The drawing under review shows one solid part. Ordinate dimensions are in mm from its lowest x, y, z. A direction names the side the tool comes from. Round coordinates to 2 decimals unless told otherwise and drop trailing zeros. Put each result on its own line as item: value. Start each with the question number.
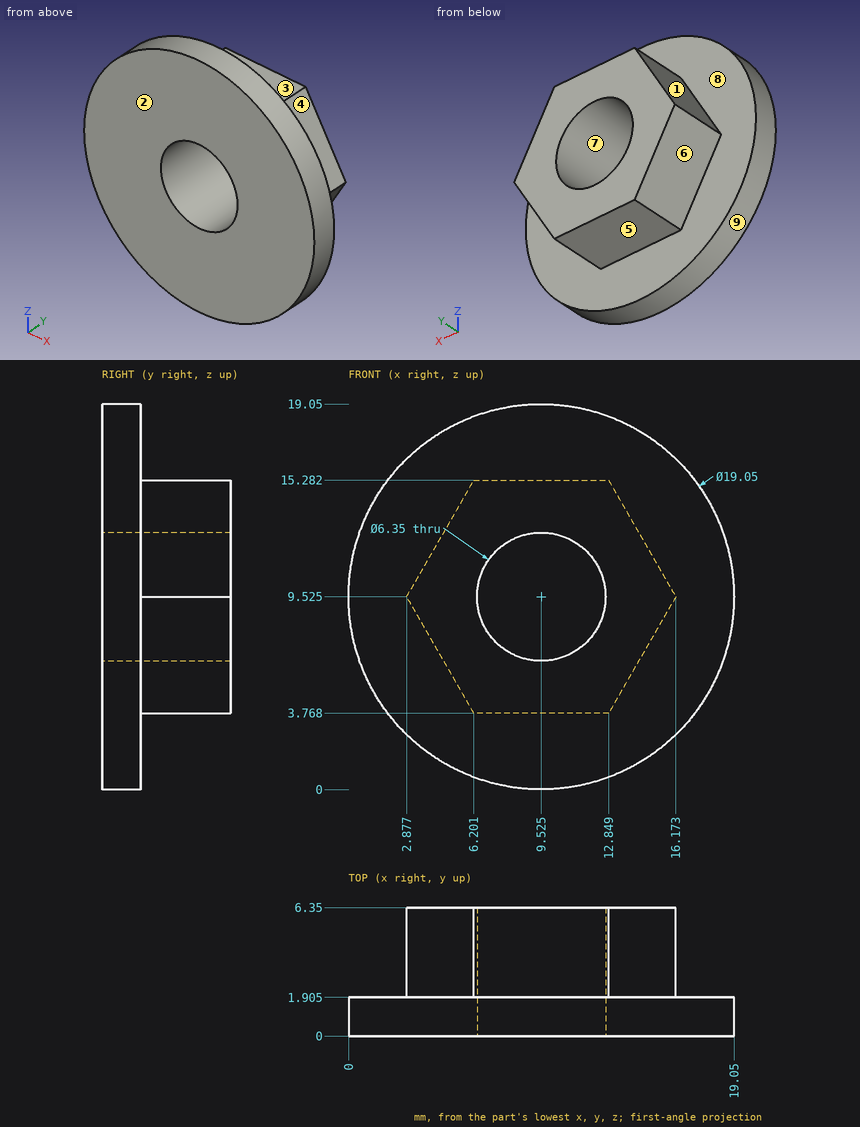
Item 1: For L1, parallel to Y at x = 15.75, z = 3.75 (1 decimal); L2, parallel to Z at x = 7, y = 1.25; L3, parallel to Z at x = 12.25, y = 6 (1 decimal), list the stretches that pass through material, from the lowest coordinate up.
Item 2: Tool access review of the marked faces 1, 2, 3, 4 and 5: name each direction out of +Z, -Z, +X, -X, +Y, -Y from which nothing blocks a thin tool from reaching the whole face with its end or side.
Item 3: Mouldability with a two-part tool opening along Z and no side actions: class the marked faces 6, 7, 8 and 9 as +Z half, -Z half, draft (parallel to the pull), parting line (faces both ways), or undercut.
Item 4: Insertion check: pin 1 Ø1.5 at (y, z) = (2, 6) entering from +X (1 decimal); pin 2 Ø3.5 at (x, y) = (10.5, 4.5) entering from +Z. Each pin has a flat end and moves straight along its axis. Give the tip position at first contact, or say it passes through.
Evaluation:
1. L1: y = 0 to 1.9
1. L2: z = 0.34 to 7.6, 11.45 to 18.71
1. L3: z = 3.8 to 7.9, 11.2 to 15.3
2. face 1: +Z, -X, +Y
2. face 2: +Z, -Z, +X, -X, -Y
2. face 3: +Z, +X, -X, +Y
2. face 4: +Z, +X, +Y
2. face 5: -Z, +X, -X, +Y
3. face 6: -Z half
3. face 7: undercut
3. face 8: draft
3. face 9: parting line
4. pin 1: stops at x = 18.6
4. pin 2: stops at z = 15.28
